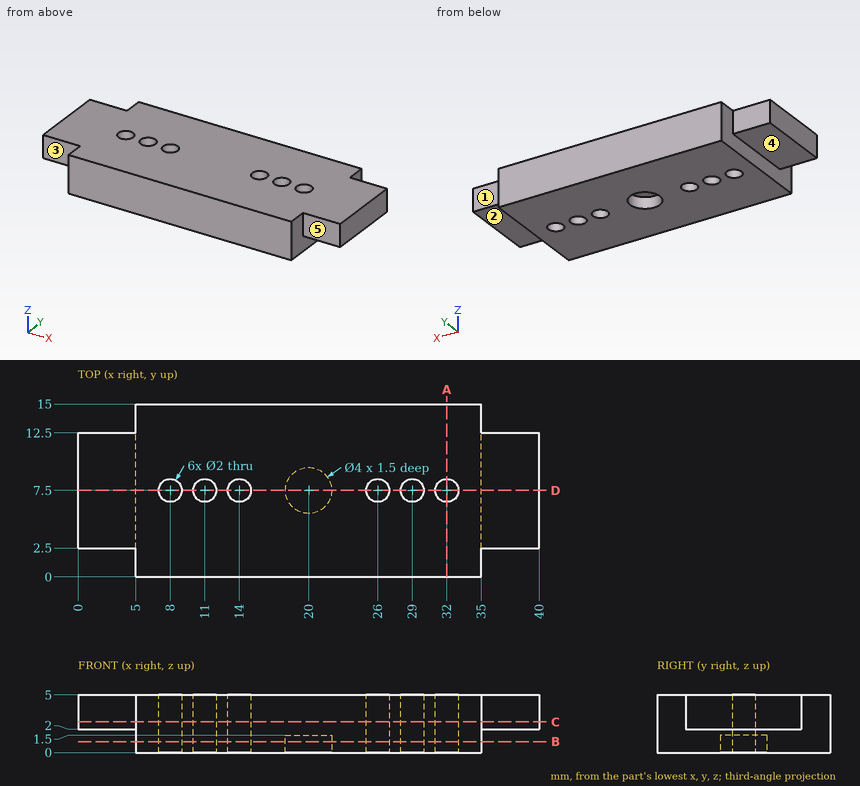
Check sheet for the drawn part. Datum: minimum x, y, z corner. Units: mm. A direction names the side the tool comes from. Round coordinates to 2 decimals unless told otherwise and drop trailing zeros. Loops run counter-clockwise (first coordinate to the right, second up) from the corner with the lowest first, then second, coordinate; pieces in that order, holes last. Notation, with made-up numbers: (-39, 21) -> (-20, 21) arc R18 cw to (-20, 29) -> close; hole circle Ø11 at (8.25, -32). An arc over 180 degrees is marked (long way). Put each result on its own line as item: value. Start each with the question number.
1. Section check C-C (z = 2.65). Enter the section's corners in (x, y).
2. Section check A-A (x = 32). Enter the section's corners in (y, z).
3. Section check D-D (y = 7.5). Give the number of separate pieces and of enclosed holes in the cut face, plus the area to 3 significant figures.
4. Gauge pin test, flat ends, axial feed: pin 1 (2.5 mm diameter, centred on x = 38.5, y = 5.5, fed in from -Z); pin 2 (1.8 mm diameter, centred on x = 29, y = 7.5, fed in from -Z); pin 3 (0.9 mm diameter, centred on x = 3.5, z = 3.5, fed in from +Y); pin 4 (0.9 mm diameter, centred on x = 37.5, z = 3, fed in from -Y). Record the tip position at first contact, or that the pin passes through.
5. Section check B-B (z = 0.95). Enter the section's corners in (x, y), plus the area to 3 significant figures.
6. Access from +Z, -Z, +X, -X, +Y, -Y to the whole of each face (thin tool, end or side, straight path). Record for the marked faces 1, 2, 3, 4 and 5.
7. Scan lines: probe 1 along Y at (x, z) = (26, 3.9); probe 2 along Y at (x, z) = (20, 0.8); probe 3 along X at (y, z) = (11.5, 1.6). Record each from-to range of solid material in increasing order.
Findings:
1. outline: (0, 2.5) -> (5, 2.5) -> (5, 0) -> (35, 0) -> (35, 2.5) -> (40, 2.5) -> (40, 12.5) -> (35, 12.5) -> (35, 15) -> (5, 15) -> (5, 12.5) -> (0, 12.5) -> close; hole circle Ø2 at (8, 7.5); hole circle Ø2 at (11, 7.5); hole circle Ø2 at (14, 7.5); hole circle Ø2 at (26, 7.5); hole circle Ø2 at (29, 7.5); hole circle Ø2 at (32, 7.5)
2. outline: (0, 0) -> (6.5, 0) -> (6.5, 5) -> (0, 5) -> close; (8.5, 0) -> (15, 0) -> (15, 5) -> (8.5, 5) -> close
3. separate pieces: 7
3. enclosed holes: 0
3. area: 114 mm^2
4. pin 1: stops at z = 2
4. pin 2: passes through
4. pin 3: stops at y = 12.5
4. pin 4: stops at y = 2.5
5. outline: (5, 0) -> (35, 0) -> (35, 15) -> (5, 15) -> close; hole circle Ø2 at (8, 7.5); hole circle Ø2 at (11, 7.5); hole circle Ø2 at (14, 7.5); hole circle Ø4 at (20, 7.5); hole circle Ø2 at (26, 7.5); hole circle Ø2 at (29, 7.5); hole circle Ø2 at (32, 7.5)
5. area: 419 mm^2
6. face 1: +Z, -Z, +X, +Y
6. face 2: -Z, +X, +Y, -Y
6. face 3: +Z, -Z, -X, -Y
6. face 4: -Z, -X, +Y, -Y
6. face 5: +Z, -Z, +X, -Y
7. probe 1: y = 0 to 6.5, 8.5 to 15
7. probe 2: y = 0 to 5.5, 9.5 to 15
7. probe 3: x = 5 to 35
